from build123d import *

# Parameters (mm, degrees)
SKETCH2_W  = 12
SKETCH2_H  = 2
SLOT_DEPTH = 3.6


with BuildPart() as part:
    # BodySke → BaseBody (revolve)
    with BuildSketch(Plane.XY, mode=Mode.PRIVATE) as basebody_sk:
        Polygon((43.7, 4.25), (50, 4.25), (50, 0), (0, 0), (0, 5.036), (0.556565659, 6), (41.95, 6), align=None)
    revolve(basebody_sk.sketch.rotate(Axis((-12.7, 0, 0), (1, 0, 0)), 90), axis=Axis((-12.7, 0, 0), (1, 0, 0)))

    # Sketch2 → Slot (cut)
    with BuildSketch(Plane(origin=(0, 0, 0), x_dir=(0, 0, -1), z_dir=(1, 0, 0))):
        Rectangle(SKETCH2_W, SKETCH2_H)
    extrude(amount=SLOT_DEPTH, mode=Mode.SUBTRACT)


solid = part.part
Geometry: final body of the model. Coordinates: model frame, mm. A direction names the side the tool comes from. Give positions to 0.01 mm unless a question says otherwise; leave off trailing zeros. Loops run counter-clockwise (first coordinate to the right, second up) from the corner with the lowest first, then second, coordinate; pieces in that order, holes last. Notation, with made-up numbers: (76.25, 7.5) -> (117.25, 7.5) arc R17 ccw to (117.25, 22.5) -> close; hole circle Ø11 at (1, 1.25). An arc over 180 degrees is marked (long way). Put each result on its own line as item: value.
1. Pin query (flat end, axial travel): P1, Ø2, axis at x = 25, z = 2.5, coming from the +Y side; P2, Ø3, axis at x = 19.5, y = -4.5, coming from the -Z side; P3, Ø5, axis at x = 33, z = -4.5, coming from the -Y side. Return the tip coordinate at first contact, or that it passes through.
Taken from the geometry:
P1: stops at y = 5.81
P2: stops at z = -5.2
P3: stops at y = -5.66
2. Cut plane A-A (y = 0). Return the cut outline in (x, z), plus the area to 3 significant figures.
Taken from the geometry:
outline: (3.6, -6) -> (41.95, -6) -> (43.7, -4.25) -> (50, -4.25) -> (50, 4.25) -> (43.7, 4.25) -> (41.95, 6) -> (3.6, 6) -> close
area: 532 mm2
3. Ray query, line 1 along Y through (x, z) = (7, 3.25); line 2 along Z through (x, y) = (8, 1.25); line 3 along Z through (x, y) = (6, 4.5). Return the intervals inside material, ascending. Write a range as [from, to].
Taken from the geometry:
line 1: y = [-5.04, 5.04]
line 2: z = [-5.87, 5.87]
line 3: z = [-3.97, 3.97]
4. Set-up query: faces 4 (the flat face through (0, -3, 0)), 5 (the cylindrical face through (46.894, -4.214, -0.553)), 6 (the flat face through (2, 1, 0)). Return all of +Z, -Z, +X, -X, +Y, -Y with unobstructed straight access to the full face (end or side cutting, diameter ignored); none if empty.
Taken from the geometry:
face 4: +Z, -Z, -X, +Y, -Y
face 5: +X
face 6: +Z, -Z, -X
5. Cut plane C-C (x = 37). Return the cut outline in (y, z).
Taken from the geometry:
outline: circle Ø12 at (0, 0)
6. Cut plane B-B (z = 0). Return the cut outline in (x, y).
Taken from the geometry:
outline: (0, -5.04) -> (0.56, -6) -> (41.95, -6) -> (43.7, -4.25) -> (50, -4.25) -> (50, 4.25) -> (43.7, 4.25) -> (41.95, 6) -> (0.56, 6) -> (0, 5.04) -> (0, 1) -> (3.6, 1) -> (3.6, -1) -> (0, -1) -> close
7. Pull-direction query (Y, two-part tool) for faces 1 (the flat face through (50, 0, 0)), 2 (the flat face through (3.6, 0, 0)), 3 (the cylindrical face through (21.543, -1.802, 5.723)); classes: released by +Y, released by -Y, zero draft, split by the parting line, or undercut.
Taken from the geometry:
face 1: zero draft
face 2: undercut
face 3: split by the parting line
